```python
from build123d import *

# Parameters (mm, degrees)
SKETCH1_R           = 11.5
BOSS_EXTRUDE1_DEPTH = 3
SKETCH2_R           = 9
BOSS_EXTRUDE2_DEPTH = 10
BOSS_EXTRUDE2_TAPER = 15
SKETCH3_R           = 2
CUT_EXTRUDE1_DEPTH  = 21.820662814


with BuildPart() as part:
    # Sketch1 → Boss-Extrude1 (new body)
    with BuildSketch(Plane.XY):
        Circle(SKETCH1_R)
    extrude(amount=BOSS_EXTRUDE1_DEPTH)

    # Sketch2 → Boss-Extrude2 (add)
    with BuildSketch(Plane.XY.offset(3)):
        Circle(SKETCH2_R)
    extrude(amount=BOSS_EXTRUDE2_DEPTH, taper=BOSS_EXTRUDE2_TAPER)

    # Sketch3 → Cut-Extrude1 (cut, through all)
    with BuildSketch(Plane.XY.offset(13)):
        Circle(SKETCH3_R)
    extrude(amount=-CUT_EXTRUDE1_DEPTH, mode=Mode.SUBTRACT)


solid = part.part
```
Can you work these out from the model? Positions are in its coordinate system, mm. A direction names the side the tool comes from. Coordinates: 2 decimals unless noted, no trailing zeros. Order: outer loops, then holes, each group sorted by start corner. A loop starts at its lowest first (then second) coordinate and runs counter-clockwise, first axis right, second up.
1. If we section it at C-C (z = 8): Please give me the cut outline in (x, y).
2. I need wall thicknesses on line 1 (Z direction, x = 9, y = -2.75); line 2 (Y direction, x = 0, z = 5.25); line 3 (Y direction, x = -1.25, z = 12.25). Which ranges of each line are inside material? Lowest first, please.
3. If we section it at D-D (z = 4.25): Please give me the cut outline in (x, y).
4. I'm going to push flat-ended pins straight in: pin 1 (4 mm diameter, centred on x = -7, z = 2.5, fed in from -Y); pin 2 (1.5 mm diameter, centred on x = -4, z = 3.5, fed in from +Y); pin 3 (2 mm diameter, centred on x = 6, z = 7, fed in from -Y). Where does each tip first touch, or does it pass through?
5. If we section it at A-A (y = 0): Please give me the cut outline in (x, z), then the cut area to 3 significant figures.
6. Thinking about a two-plate mould opening in Y: for faces 3 (the face through (-0.2, -2.4, 0)), 4 (the face through (-1.5, 11.4, 1.5)), 5 (the face through (0, -2, 7)), which applies, +Y half, -Y half, draft (parallel to the pull), parting line (faces both ways), or undercut?
7. For faces 1 (the face through (0, -3, 13)), 2 (the face through (-7, -6, 3)), which set-ups out of +Z, -Z, +X, -X, +Y, -Y let a thin tool reach every point of the face, with its end or its side?
Entries:
1. outline: circle Ø15.32 at (0, 0); hole circle Ø4 at (0, 0)
2. line 1: z = 0 to 3
2. line 2: y = -8.4 to -2, 2 to 8.4
2. line 3: y = -6.4 to -1.56, 1.56 to 6.4
3. outline: circle Ø17.33 at (0, 0); hole circle Ø4 at (0, 0)
4. pin 1: stops at y = -10.36
4. pin 2: stops at y = 10.97
4. pin 3: stops at y = -6.22
5. outline: (-11.5, 0) - (-2, 0) - (-2, 13) - (-6.32, 13) - (-9, 3) - (-11.5, 3) - close; (2, 0) - (11.5, 0) - (11.5, 3) - (9, 3) - (6.32, 13) - (2, 13) - close
5. area: 170 mm2
6. face 3: draft
6. face 4: parting line
6. face 5: undercut
7. face 1: +Z, +X, -X, +Y, -Y
7. face 2: +Z
